from build123d import *

# Parameters (mm, degrees)
CUT_EXTRUDE1_DEPTH      = 1
CUT_EXTRUDE1_DEPTH_BACK = 40


with BuildPart() as part:
    # Sketch1 → Revolve1 (revolve)
    with BuildSketch(Plane.XY):
        Polygon((-6.35, 0), (-8.35, 0), (-8.35, 39), (0, 39), (0, 37), (-4.35, 37), (-4.35, 21), (-6.35, 21), align=None)
    revolve(axis=Axis((0, 0, 0), (0, 1, 0)))

    # Sketch2 → Cut-Extrude1 (cut, two sides)
    with BuildSketch(Plane(origin=(0, 39, 0), x_dir=(1, 0, 0), z_dir=(0, 1, 0))) as cut_extrude1_sk:
        Polygon((-0.65, 0.65), (-7, 0.65), (-11.662246707, 0.65), (-11.662246707, -0.65), (-7, -0.65), (-0.65, -0.65), (-0.65, -7), (0.65, -7), (0.65, -0.65), (7, -0.65), (7, 0.65), (0.65, 0.65), (0.65, 7), (-0.65, 7), align=None)
    extrude(amount=CUT_EXTRUDE1_DEPTH, mode=Mode.SUBTRACT)
    extrude(cut_extrude1_sk.sketch, amount=-CUT_EXTRUDE1_DEPTH_BACK, mode=Mode.SUBTRACT)


solid = part.part
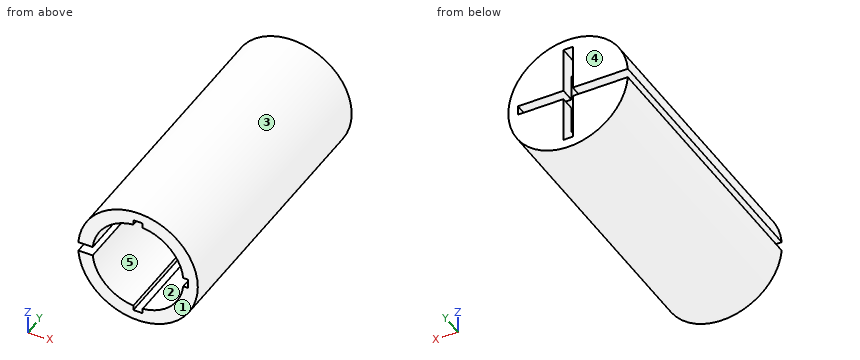
CAD build for the part. Positions are in the model's coordinates, mm. Face numbers are marked on the shaded views. A direction names the side the tool comes from. Round coordinates to 2 decimals unless told otherwise and drop trailing zeros. Loops run counter-clockwise (first coordinate to the right, second up) from the corner with the lowest first, then second, coordinate; pieces in that order, holes last. Notation, with made-up numbers: M 82.5,14.5 L 122.5,14.5 A15 ccw 122.5,21.5 Z; hole C 85,54 d9. An arc over 180 degrees is marked long. One line per question, with ' | ' between items. Start each with the question number.
Item 1: Which spindle directions (+Z, -Z, +X, -X, +Y, -Y) get a long thin tool onto all of the face, cutting with end or side? Do the marked faces 1 and 2. Say none if no direction does.
Item 2: Two-plate mould, pull along X, no slides. Class the marked faces 3, 4 and 5: pulls with the +X half, pulls with the -X half, needs draft (parallel to the pull), parting line crosses it, or undercut.
Item 3: Pin check, flat tips, straight feed: pin 1 Ø1.5 at (x, y) = (-2.5, 34.5) entering from -Z; pin 2 Ø6 at (x, y) = (-3, 26.5) entering from +Z; pin 3 Ø7 at (y, z) = (11.5, -5) entering from -X; pin 4 Ø2 at (y, z) = (10, -5.5) entering from -X. Stop position of each tip, or through.
Item 4: Cut at D-D, the plane x = -3.5. Write the cut outline in (y, z).
Item 5: Cut at C-C, the plane y = 28. Write the cut outline in (x, z).
Item 6: Wall check: line 1 (Z direction, x = 0.25, y = 22.5); line 2 (X direction, y = 34.5, z = 0.25); line 3 (Y direction, x = -5, z = -3). Give the ranges that are in metal, low to high.
Item 7: Cut at A-A, the plane x = 0. Write the cut outline in (y, z), plus the area to 3 significant figures.
Item 8: Cut at B-B, the plane z = 5. Write the cut outline in (x, y).
Responses:
1) face 1: +Z, -Z, +X, -X, -Y | face 2: -Y
2) face 3: parting line crosses it | face 4: needs draft | face 5: undercut
3) pin 1: stops at z = -8.16 | pin 2: stops at z = 8.35 | pin 3: stops at x = -8.21 | pin 4: stops at x = -7.03
4) outline: M 0,-7.58 L 39,-7.58 L 39,-0.65 L 37,-0.65 L 37,-2.58 L 21,-2.58 L 21,-5.3 L 0,-5.3 Z; M 0,5.3 L 21,5.3 L 21,2.58 L 37,2.58 L 37,0.65 L 39,0.65 L 39,7.58 L 0,7.58 Z
5) outline: M -8.32,-0.65 A8.35 ccw long -8.32,0.65 L -4.3,0.65 A4.35 cw -0.65,4.3 L -0.65,7 L 0.65,7 L 0.65,4.3 A4.35 cw 4.3,0.65 L 7,0.65 L 7,-0.65 L 4.3,-0.65 A4.35 cw 0.65,-4.3 L 0.65,-7 L -0.65,-7 L -0.65,-4.3 A4.35 cw -4.3,-0.65 Z
6) line 1: z = -8.35 to -7, 7 to 8.35 | line 2: x = 7 to 8.35 | line 3: y = 21 to 39
7) outline: M 0,-8.35 L 39,-8.35 L 39,-7 L 0,-7 Z; M 0,7 L 39,7 L 39,8.35 L 0,8.35 Z | area: 105 mm²
8) outline: M -6.69,0 L -3.91,0 L -3.91,21 L -0.65,21 L -0.65,39 L -6.69,39 Z; M 0.65,21 L 3.91,21 L 3.91,0 L 6.69,0 L 6.69,39 L 0.65,39 Z
